Check sheet for the modelled part. Datum: model origin and axes. Units: mm. Face numbers are marked on the shaded views. Give positions to 0.01 mm unless a question says otherwise; leave off trailing zeros. Loops run counter-clockwise (first coordinate to the right, second up) from the corner with the lowest first, then second, coordinate; pieces in that order, holes last. Notation, with made-up numbers: (-2.5, -20.75) - (14.5, -20.75) arc R24 ccw to (14.5, -4.75) - close; hole circle Ø8 at (-14, -17). An arc over 180 degrees is marked (long way). Answer in a Markdown table with one row per item. Add a question column.
(1) Go/stop test with flat-tipped pins: P1, Ø6, axis at x = -75.5, z = -245.5, coming from the -Y side; P2, Ø3, axis at x = -70, z = -25, coming from the -Y side; P3, Ø12.5, axis at x = 169.5, z = -33.5, coming from the -Y side. Record where each tip stops, or that it passes through.
(2) Thickness scan on L1, parallel to Z at x = 0, y = -7.5; L2, parallel to Z at x = 0, y = 40; L3, parallel to X at y = 19.5, z = 0. Record the ranges inside material, lowest first.
(3) Sectioned sample at A-A on y = 600. Enter the section's corners in (x, z).
(4) Sectioned sample at D-D on y = 407. Enter the section's corners in (x, z), then the cut area to 3 significant figures.
(5) Sectioned sample at C-C on z = 0. Enter the section's corners in (x, y).
(6) Draft check along Z on the marked faces 1, 2 and 3. Enter one of: released by +Z, released by -Z, zero draft, split by the parting line, or undercut.
(7) Sectioned sample at B-B on x = 372.5. Enter the section's corners in (y, z), then the cut area to 3 significant figures.
from build123d import *

# Parameters (mm, degrees)
F0_W      = 193.3809220791
F0_H      = 196.0519328713
F0_R      = 74.8892897361
F1_DEPTH  = 25.4
F2_W      = 193.3809220791
F2_H      = 196.0519328713
F2_R      = 74.655991807
F3_DEPTH  = 25.4
F4_W      = 176.1402115226
F4_H      = 196.0519328713
F4_R      = 74.3860816692
F4_W_2    = 17.2407105565
F5_DEPTH  = 25.4
F6_W      = 193.3809220791
F6_H      = 196.0519328713
F6_R      = 75.3545401658
F7_DEPTH  = 25.4
F8_W      = 193.4532523155
F8_H      = 35.7192189813
F9_DEPTH  = 25.4
F11_DEPTH = 404.6249985695
F12_W     = 1055.474460125
F12_H     = 918.9680218697
F13_DEPTH = 25.4
F14_W     = 752.8154850006
F14_H     = 912.7593636513
F15_DEPTH = 25.4
F16_W     = 870.2914460182
F16_H     = 272.9075178504
F17_DEPTH = 25.4
F18_W     = 400.6907343864
F18_H     = 395.6300988793
F19_DEPTH = 25.4
F20_W     = 571.7930793762
F20_H     = 567.36561656
F21_DEPTH = 25.4
F23_W     = 78.0102312565
F23_H     = 34.4761013985
F23_W_2   = 13.3122801781
F23_H_2   = 332.7346146107
F23_W_3   = 187.4931752682
F23_H_3   = 105.7706475258
F23_H_4   = 99.6497869492
F24_DEPTH = 25.4
F25_W     = 101.5389561653
F25_H     = 251.5766620636
F25_H_2   = 50.2630472183
F25_W_2   = 29.5691788197
F25_W_3   = 54.5960366726
F25_H_3   = 76.733738184
F26_DEPTH = 25.4


with BuildPart() as f1:
    # F0 (on Front) → F1 (new body)
    with BuildSketch(Plane.XZ):
        with Locations((-0.0024288893, -0.3737099469)):
            Rectangle(F0_W, F0_H)
        Circle(F0_R, mode=Mode.SUBTRACT)
    extrude(amount=F1_DEPTH)

    # F2 (on face) → F3 (join)
    with BuildSketch(Plane(origin=(0, 0, 0), x_dir=(-1, 0, 0), z_dir=(0, 1, 0))):
        with Locations((0.0024288893, -0.3737099469)):
            Rectangle(F2_W, F2_H)
        Circle(F2_R, mode=Mode.SUBTRACT)
    extrude(amount=F3_DEPTH)

    # F4 (on face) → F5 (join)
    with BuildSketch(Plane(origin=(0, 25.4, 0), x_dir=(-1, 0, 0), z_dir=(0, 1, 0))):
        with Locations((-8.617926389, -0.3737099469)):
            Rectangle(F4_W, F4_H)
        Circle(F4_R, mode=Mode.SUBTRACT)
        with Locations((88.0725346506, -0.3737099469)):
            Rectangle(F4_W_2, F4_H)
    extrude(amount=F5_DEPTH)

    # F6 (on face) → F7 (join)
    with BuildSketch(Plane.XZ.offset(25.4)):
        with Locations((-0.0024288893, -0.3737099469)):
            Rectangle(F6_W, F6_H)
        Circle(F6_R, mode=Mode.SUBTRACT)
    extrude(amount=F7_DEPTH)

    # F8 (on face) → F9 (join)
    with BuildSketch(Plane(origin=(0, 0, -98.3996763825), x_dir=(1, 0, 0), z_dir=(0, 0, -1))):
        with Locations((0.0337362289, 68.6596094906)):
            Rectangle(F8_W, F8_H)
        Polygon((96.7603623867, 50.8), (-96.6928899288, 50.8), (-97.9034900665, 50.8), (-97.9034900665, -97.2673520446), (96.7603623867, -97.2673520446), align=None)
    extrude(amount=F9_DEPTH)

    # F10 (on face) → F11 (join)
    with BuildSketch(Plane(origin=(0, 50.8, 0), x_dir=(-1, 0, 0), z_dir=(0, 1, 0))):
        Polygon((-65.7769590616, -350.3327965736), (-65.7769590616, -371.3071942329), (119.0916895866, -371.3071942329), (119.0916895866, -98.3996763825), (-65.7769590616, -98.3996763825), align=None)
    extrude(amount=F11_DEPTH)

    # F12 (on face) → F13 (join)
    with BuildSketch(Plane.XY.offset(-98.3996763825)):
        with Locations((-85.7326686382, 188.2182061672)):
            Rectangle(F12_W, F12_H)
    extrude(amount=F13_DEPTH)

    # F14 (on face) → F15 (join)
    with BuildSketch(Plane(origin=(0, 0, -371.3071942329), x_dir=(1, 0, 0), z_dir=(0, 0, -1))):
        with Locations((42.0474410057, -250.8960068226)):
            Rectangle(F14_W, F14_H)
    extrude(amount=F15_DEPTH)

    # F16 (on face) → F17 (join)
    with BuildSketch(Plane.YZ.offset(65.7769590616)):
        with Locations((20.2792755604, -234.8534353077)):
            Rectangle(F16_W, F16_H)
    extrude(amount=F17_DEPTH)

    # F18 (on face) → F19 (join)
    with BuildSketch(Plane(origin=(65.7769590616, 0, 0), x_dir=(0, -1, 0), z_dir=(-1, 0, 0))):
        with Locations((176.6569912434, -232.9259328544)):
            Rectangle(F18_W, F18_H)
    extrude(amount=F19_DEPTH)

    # F20 (on face) → F21 (join)
    with BuildSketch(Plane.XY.offset(-72.9996763825)):
        with Locations((-88.7070894241, 187.6235455275)):
            Rectangle(F20_W, F20_H)
        Polygon((40.3769590616, -50.8), (-18.691013125, -50.8), (-18.691013125, 275.1325964928), (-18.691013125, 292.6656007767), (40.3769590616, 292.6656007767), (164.7324860096, 292.6656007767), (164.7324860096, -50.8), (129.8503279686, -50.8), align=None, mode=Mode.SUBTRACT)
    extrude(amount=F21_DEPTH)

    # F23 (on face) → F24 (join)
    with BuildSketch(Plane.XY.offset(-47.5996763825)):
        Polygon((119.2969679832, -40.3836667538), (119.2969679832, 292.3509478569), (-242.377102375, 292.3509478569), (-242.377102375, -40.3836667538), (-68.1962072849, -40.3836667538), align=None)
        with Locations((158.3020836115, 309.5889985561)):
            Rectangle(F23_W, F23_H)
        Polygon((-242.377102375, 292.3509478569), (119.2969679832, 292.3509478569), (119.2969679832, 326.8270492554), (-389.0109658241, 326.8270492554), (-389.0109658241, 292.3509478569), (-255.6893825531, 292.3509478569), align=None)
        with Locations((-249.0332424641, 125.9836405516)):
            Rectangle(F23_W_2, F23_H_2)
        with Locations((25.5503803492, -93.2689905167)):
            Rectangle(F23_W_3, F23_H_3)
        with Locations((-249.0332424641, -90.2085602283)):
            Rectangle(F23_W_2, F23_H_4)
    extrude(amount=F24_DEPTH)

    # F25 (on face) → F26 (join)
    with BuildSketch(Plane.XY.offset(-47.5996763825)):
        Polygon((101.5389561653, 0), (0, 0), (-69.8948949575, 0), (-69.8948949575, -46.3175177574), (101.5389561653, -46.3175177574), align=None)
        Polygon((-69.8948949575, 0), (0, 0), (0, 251.5766620636), (0, 301.8397092819), (-69.8948949575, 301.8397092819), (-69.8948949575, 239.4688427448), align=None)
        with Locations((50.7694780827, 125.7883310318)):
            Rectangle(F25_W, F25_H)
        Polygon((-69.8948949575, -46.3175177574), (-69.8948949575, 0), (-69.8948949575, 239.4688427448), (-116.5921464562, 239.4688427448), (-116.5921464562, -46.3175177574), (-88.026702404, -46.3175177574), align=None)
        with Locations((50.7694780827, 276.7081856728)):
            Rectangle(F25_W, F25_H_2)
        Polygon((-116.5921464562, 239.4688427448), (-69.8948949575, 239.4688427448), (-69.8948949575, 301.8397092819), (-248.7161755562, 301.8397092819), (-248.7161755562, 239.4688427448), align=None)
        with Locations((116.3235455751, 276.7081856728)):
            Rectangle(F25_W_2, F25_H_2)
        Polygon((-116.5921464562, -46.3175177574), (-116.5921464562, 239.4688427448), (-248.7161755562, 239.4688427448), (-248.7161755562, -46.3175177574), (-194.1201388836, -46.3175177574), (-182.6541610062, -46.3175177574), align=None)
        Polygon((-88.026702404, -120.3344464302), (-88.026702404, -46.3175177574), (-116.5921464562, -46.3175177574), (-182.6541610062, -46.3175177574), (-182.6541610062, -120.3344464302), align=None)
        with Locations((-221.4181572199, -84.6843868494)):
            Rectangle(F25_W_3, F25_H_3)
    extrude(amount=F26_DEPTH)


solid = f1.part
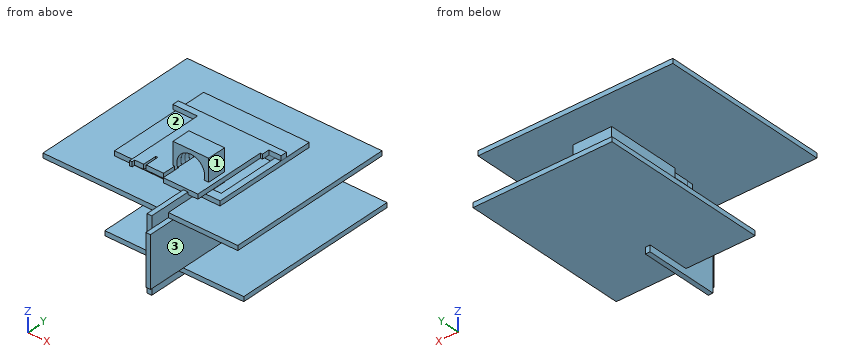
Reply:
| question | item | result |
|---|---|---|
| 1 | P1 | y = 50.8 |
| 1 | P2 | y = -50.8 |
| 1 | P3 | y = 292.35 |
| 2 | L1 | -396.71 to -371.31, -123.8 to -73, -47.6 to -22.2, 74.89 to 97.65 |
| 2 | L2 | -396.71 to -371.31, -123.8 to -73, -47.6 to -22.2, 74.39 to 97.65 |
| 2 | L3 | -96.69 to -74.66, 74.66 to 96.69 |
| 3 | outline | (-613.47, -98.4) - (442, -98.4) - (442, -73) - (-613.47, -73) - close; (-334.36, -396.71) - (418.46, -396.71) - (418.46, -371.31) - (-334.36, -371.31) - close |
| 4 | outline | (-613.47, -98.4) - (-119.09, -98.4) - (-119.09, -371.31) - (-334.36, -371.31) - (-334.36, -396.71) - (418.46, -396.71) - (418.46, -371.31) - (91.18, -371.31) - (91.18, -98.4) - (442, -98.4) - (442, -73) - (197.19, -73) - (197.19, -47.6) - (-374.6, -47.6) - (-374.6, -73) - (-613.47, -73) - close |
| 4 | area | 118,000 mm^2 |
| 5 | outline | (-96.69, -50.8) - (-75.35, -50.8) - (-75.35, -25.4) - (-74.89, -25.4) - (-74.89, 0) - (-74.66, 0) - (-74.66, 25.4) - (-74.39, 25.4) - (-74.39, 50.8) - (-96.69, 50.8) - close; (74.39, 25.4) - (74.66, 25.4) - (74.66, 0) - (74.89, 0) - (74.89, -25.4) - (75.35, -25.4) - (75.35, -50.8) - (96.69, -50.8) - (96.69, 50.8) - (74.39, 50.8) - close |
| 6 | face 1 | zero draft |
| 6 | face 2 | released by +Z |
| 6 | face 3 | undercut |
| 7 | outline | (-271.27, -98.4) - (647.7, -98.4) - (647.7, -73) - (-271.27, -73) - close; (-205.48, -396.71) - (707.28, -396.71) - (707.28, -371.31) - (-205.48, -371.31) - close |
| 7 | area | 46,500 mm^2 |
